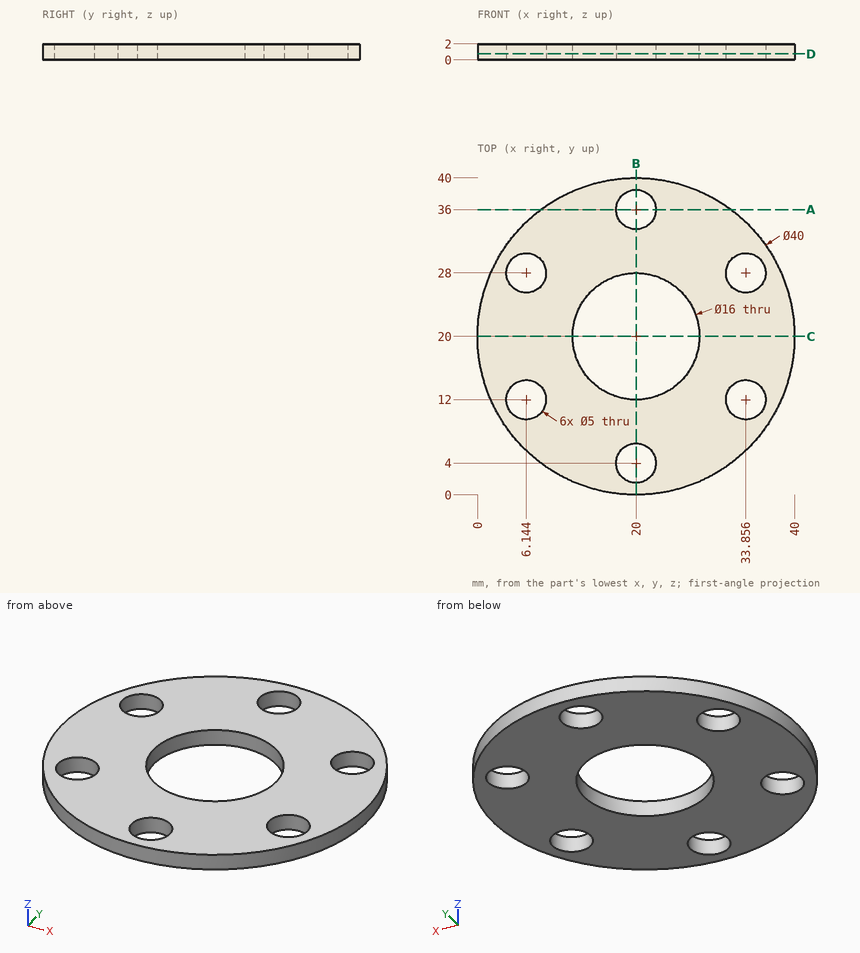
Geometry: see drawing. Coordinates: mm, zero at the bounding-box minimum. Coordinates: 2 decimals unless noted, no trailing zeros. Write each loop counter-clockwise with the first axis right and the second up, starting at its lowest first coordinate (ties: lowest second). Pieces come first, ordered by that corner, then holes.
1) Section A-A on y = 36. Output: boundary loops of the cut face in (x, z), and give its area (3 significant figures).
2) Section B-B on x = 20. Output: boundary loops of the cut face in (y, z), and give its area (3 significant figures).
3) Material intervals for line 1 along X through (y, z) = (20, 1.15); line 2 along X through (y, z) = (10.5, 1.9) (1 decimal); line 3 along Y through (x, z) = (5.5, 0.45) (1 decimal), sorted ascending.
4) Section D-D on z = 0.75. Output: boundary loops of the cut face in (x, y).
5) Section C-C on y = 20. Output: boundary loops of the cut face in (x, z).
Check result:
1. outline: (8, 0) - (17.5, 0) - (17.5, 2) - (8, 2) - close; (22.5, 0) - (32, 0) - (32, 2) - (22.5, 2) - close
1. area: 38.0 mm2
2. outline: (0, 0) - (1.5, 0) - (1.5, 2) - (0, 2) - close; (6.5, 0) - (12, 0) - (12, 2) - (6.5, 2) - close; (28, 0) - (33.5, 0) - (33.5, 2) - (28, 2) - close; (38.5, 0) - (40, 0) - (40, 2) - (38.5, 2) - close
2. area: 28.0 mm2
3. line 1: x = 0 to 12, 28 to 40
3. line 2: x = 2.4 to 4.1, 8.1 to 31.9, 35.9 to 37.6
3. line 3: y = 6.2 to 9.6, 14.4 to 25.6, 30.4 to 33.8
4. outline: circle Ø40 at (20, 20); hole circle Ø5 at (6.14, 12); hole circle Ø5 at (6.14, 28); hole circle Ø16 at (20, 20); hole circle Ø5 at (20, 4); hole circle Ø5 at (20, 36); hole circle Ø5 at (33.86, 12); hole circle Ø5 at (33.86, 28)
5. outline: (0, 0) - (12, 0) - (12, 2) - (0, 2) - close; (28, 0) - (40, 0) - (40, 2) - (28, 2) - close
